Can you work these out from the model? Positions are in its coordinate system, mm. A direction names the side the tool comes from. Round coordinates to 2 decimals unless told otherwise and drop trailing zeros. Write each loop counter-clockwise with the first axis right and the second up, starting at its lowest first coordinate (ties: lowest second). Pieces come first, ordered by that corner, then holes. Notation, with made-up numbers: (62, 74) -> (74, 74) arc R21 ccw to (74, 88) -> close; hole circle Ø3 at (-8.5, 29). An arc over 180 degrees is marked (long way). Write item = value, one per line. Start each with the question number.
1) Imagine slicing it at D-D, the plane y = 44.5. Please give me the cut outline in (x, z), then the cut area to 3 significant figures.
2) I'm going to push flat-ended pins straight in: pin 1 (2.5 mm diameter, centred on y = 74.6, z = 10.5, fed in from -X); pin 2 (3.5 mm diameter, centred on x = 1, z = 10.5, fed in from -Y); pin 3 (4 mm diameter, centred on x = 0.5, y = 63, fed in from +Z); pin 4 (3 mm diameter, centred on y = 4, z = 3, fed in from -X). Where does each tip first touch, or does it pass through?
3) If I drill on line 1 (Y direction, x = 0.3, z = 10.5); line 2 (Z direction, x = -0.8, y = 74.6); line 3 (Z direction, x = -1.5, y = 35), over which ranges is the centre line in solid material (lowest first)?
4) Imagine slicing it at B-B, the plane y = 74.6. Please give me the cut outline in (x, z), then the cut area to 3 significant figures.
5) Imagine slicing it at A-A, the plane z = 10.5. Please give me the cut outline in (x, y).
6) Thinking about a two-plate mould opening in Y: for faces 4 (the face through (-2, 70, 11)), 5 (the face through (-0.03, 77.53, 7.6)), 6 (the face through (1.126, 5.082, 3.563)), 7 (the face through (0, 73, 10.9)), which applies, +Y half, -Y half, draft (parallel to the pull), parting line (faces both ways), or undercut?
7) Imagine slicing it at C-C, the plane y = 4. Please give me the cut outline in (x, z).
8) For faces 1 (the face through (0, 78.1, 11)), 2 (the face through (-2.42, 3.28, 0.73)), 3 (the face through (0, 64, 11)), which set-ups out of +Z, -Z, +X, -X, +Y, -Y let a thin tool reach every point of the face, with its end or its side?
from build123d import *

# Parameters (mm, degrees)
SKETCH1_W                                      = 7
SKETCH1_H                                      = 14
BOSS_EXTRUDE1_DEPTH                            = 70
CBORE_FOR_2_SOCKET_HEAD_CAP_SCREW1_D           = 2.4384
CBORE_FOR_2_SOCKET_HEAD_CAP_SCREW1_CBORE_D     = 4.7625
CBORE_FOR_2_SOCKET_HEAD_CAP_SCREW1_CBORE_DEPTH = 2.1844
CUT_EXTRUDE2_DEPTH                             = 71.696534569
LPATTERN1_COUNT                                = 3
LPATTERN1_PITCH                                = 2.5
LPATTERN1_COL_COUNT                            = 3
LPATTERN1_COL_PITCH                            = 2.5
FILLET1_R                                      = 0.2
CHAMFER1_SIZE                                  = 0.7
FILLET2_R                                      = 1
CUT_EXTRUDE4_DEPTH                             = 71.436141406
CUT_EXTRUDE4_DEPTH_BACK                        = 71.436141406
SKETCH6_W                                      = 1.5
SKETCH6_H                                      = 4
CHAMFER2_SIZE                                  = 0.5
FILLET4_R                                      = 0.5
SKETCH7_W                                      = 7
SKETCH7_H                                      = 14.1
BOSS_EXTRUDE2_DEPTH                            = 2
CUT_EXTRUDE5_REACH                             = 81.535
SKETCH9_R                                      = 1.65
FILLET5_R                                      = 2


with BuildPart() as part:
    # Sketch1 → Boss-Extrude1 (new body)
    with BuildSketch(Plane(origin=(0, 0, 0), x_dir=(1, 0, 0), z_dir=(0, 1, 0))):
        Rectangle(SKETCH1_W, SKETCH1_H)
    extrude(amount=BOSS_EXTRUDE1_DEPTH)

    # CBORE for #2 Socket Head Cap Screw1 (through all)
    with Locations(Plane(origin=(-3.5, 0, 0), x_dir=(0, 0, -1), z_dir=(-1, 0, 0))):
        with Locations((-3, -4), (3, -4)):
            CounterBoreHole(CBORE_FOR_2_SOCKET_HEAD_CAP_SCREW1_D / 2, CBORE_FOR_2_SOCKET_HEAD_CAP_SCREW1_CBORE_D / 2, CBORE_FOR_2_SOCKET_HEAD_CAP_SCREW1_CBORE_DEPTH)

    # Sketch4 → Cut-Extrude2 (cut, through all)
    with BuildSketch(Plane(origin=(3.5, 0, 0), x_dir=(0, 0, -1), z_dir=(1, 0, 0))):
        with BuildLine():
            Line((0.9, 220.888750438), (0.9, 70))
            ThreePointArc((0.9, 70), (0, 69.1), (-0.9, 70))
            Line((-0.9, 70), (-0.9, 220.888750438))
            Line((-0.9, 220.888750438), (-0.9, 522.666251314))
            Line((-0.9, 522.666251314), (0.9, 522.666251314))
            Line((0.9, 522.666251314), (0.9, 220.888750438))
        make_face()
    cut_extrude2 = extrude(amount=-CUT_EXTRUDE2_DEPTH, mode=Mode.SUBTRACT)

    # LPattern1: Cut-Extrude2 ×3
    with Locations(*[(0, 0, i * LPATTERN1_PITCH) for i in range(1, LPATTERN1_COUNT)]):
        add(cut_extrude2, mode=Mode.SUBTRACT)

    # LPattern1 col: Cut-Extrude2 ×3
    with Locations(*[(0, 0, -i * LPATTERN1_COL_PITCH) for i in range(1, LPATTERN1_COL_COUNT)]):
        add(cut_extrude2, mode=Mode.SUBTRACT)

    # Fillet1
    fillet1_edges = [part.edges().sort_by_distance(p)[0] for p in [
        (0, 70, -0.9),
        (0, 70, 0.9),
        (3.5, 69.1, 0),
        (-3.5, 69.1, 0),
        (0, 70, -3.4),
        (0, 70, -1.6),
        (3.5, 69.1, -2.5),
        (-3.5, 69.1, -2.5),
        (0, 70, -5.9),
        (0, 70, -4.1),
        (3.5, 69.1, -5),
        (-3.5, 69.1, -5),
        (0, 70, 1.6),
        (0, 70, 3.4),
        (3.5, 69.1, 2.5),
        (-3.5, 69.1, 2.5),
        (0, 70, 4.1),
        (0, 70, 5.9),
        (3.5, 69.1, 5),
        (-3.5, 69.1, 5),
    ]]
    fillet(fillet1_edges, radius=FILLET1_R)

    # Chamfer1
    chamfer1_edges = [part.edges().sort_by_distance(p)[0] for p in [
        (0, 70, -7),
    ]]
    chamfer(chamfer1_edges, length=CHAMFER1_SIZE)

    # Fillet2
    # the kernel refuses this fillet: 1 mm, written as the material it takes off along each edge
    with BuildSketch(Plane(origin=(-4.535533906, 69.3, -7), x_dir=(0, 0.707106781186555, 0.70710678118654), z_dir=(1, 0, 0))) as fillet2_piece_1:
        with BuildLine():
            CenterArc((FILLET2_R * 0.414213562373, FILLET2_R), FILLET2_R, 225, 45)
            Line((-FILLET2_R * 0.292893218813, FILLET2_R * 0.292893218813), (-FILLET2_R * 0.307035354437, FILLET2_R * 0.27875108319))
            Line((-FILLET2_R * 0.307035354437, FILLET2_R * 0.27875108319), (-FILLET2_R * 0.00828427124746, -FILLET2_R * 0.02))
            Line((-FILLET2_R * 0.00828427124746, -FILLET2_R * 0.02), (FILLET2_R * 0.414213562373, -FILLET2_R * 0.02))
            Line((FILLET2_R * 0.414213562373, -FILLET2_R * 0.02), (FILLET2_R * 0.414213562373, 0))
        make_face()
    extrude(amount=9.071067812, mode=Mode.SUBTRACT)
    with BuildSketch(Plane(origin=(-4.448522012, 70, -6.3), x_dir=(0, 0, 1), z_dir=(1, 0, 0))) as fillet2_piece_2:
        with BuildLine():
            CenterArc((0.438824243, 0.97538932), FILLET2_R, 225, 32.262207343)
            Line((-0.268282539, 0.268282539), (-0.282424674, 0.254140403))
            Line((-0.282424674, 0.254140403), (-0.014142136, -0.014142136))
            Line((-0.014142136, -0.014142136), (0, -0.02))
            ThreePointArc((0, -0.02), (0.109167309, -0.02), (0.213924825, -0.019507786))
            Line((0.213924825, -0.019507786), (0.218334617, 0))
        make_face()
    extrude(amount=8.897044023, mode=Mode.SUBTRACT)

    # Sketch6 → Cut-Extrude4 (cut, two sides: drawn at the far end of the back side and taken through both)
    with BuildSketch(Plane(origin=(0, 0, 0), x_dir=(0, 0, -1), z_dir=(1, 0, 0)).offset(-CUT_EXTRUDE4_DEPTH_BACK)):
        with Locations((6.25, 65)):
            Rectangle(SKETCH6_W, SKETCH6_H)
    extrude(amount=CUT_EXTRUDE4_DEPTH + CUT_EXTRUDE4_DEPTH_BACK, mode=Mode.SUBTRACT)

    # Chamfer2
    chamfer2_edges = [part.edges().sort_by_distance(p)[0] for p in [
        (0, 67, -7),
    ]]
    chamfer(chamfer2_edges, length=CHAMFER2_SIZE)

    # Fillet4
    fillet4_edges = [part.edges().sort_by_distance(p)[0] for p in [
        (0, 63, -7),
        (0, 63, -5.5),
        (0, 67.5, -7),
        (0, 67, -6.5),
    ]]
    fillet(fillet4_edges, radius=FILLET4_R)

    # Sketch7 → Boss-Extrude2 (add, symmetric)
    with BuildSketch(Plane(origin=(0, 0, 0), x_dir=(0, 0, -1), z_dir=(1, 0, 0))):
        with Locations((-10.5, 71.05)):
            Rectangle(SKETCH7_W, SKETCH7_H)
    extrude(amount=BOSS_EXTRUDE2_DEPTH, both=True)

    # Sketch9 → Cut-Extrude5 (cut, up to next)
    with BuildSketch(Plane(origin=(2, 0, 0), x_dir=(0, 0, -1), z_dir=(1, 0, 0)), mode=Mode.PRIVATE) as cut_extrude5_sk1:
        with Locations((-10.5, 74.6)):
            Circle(SKETCH9_R)
    cut_extrude5_tool1 = extrude(cut_extrude5_sk1.sketch, amount=-CUT_EXTRUDE5_REACH, mode=Mode.PRIVATE) & part.part
    add(cut_extrude5_tool1.solids().sort_by_distance((2, 74.6, 10.5))[0], mode=Mode.SUBTRACT)

    # Fillet5
    fillet5_edges = [part.edges().sort_by_distance(p)[0] for p in [
        (0, 78.1, 7),
        (0, 64, 7),
        (0, 64, 14),
        (0, 78.1, 14),
    ]]
    fillet(fillet5_edges, radius=FILLET5_R)


solid = part.part
Reported:
q1.outline = (-3.5, -7) -> (3.5, -7) -> (3.5, 7) -> (-3.5, 7) -> close
q1.area = 98.0 mm²
q2.pin_1 = through
q2.pin_2 = 63.98
q2.pin_3 = 13.73
q2.pin_4 = -1.32
q3.line_1 = 64 to 72.95, 76.25 to 78.1
q3.line_2 = 7 to 8.85, 12.15 to 14
q3.line_3 = -7 to 7
q4.outline = (-2, 7) -> (2, 7) -> (2, 8.85) -> (-2, 8.85) -> close; (-2, 12.15) -> (2, 12.15) -> (2, 14) -> (-2, 14) -> close
q4.area = 14.8 mm²
q5.outline = (-2, 64) -> (2, 64) -> (2, 72.95) -> (-2, 72.95) -> close; (-2, 76.25) -> (2, 76.25) -> (2, 78.1) -> (-2, 78.1) -> close
q6.face_4 = draft
q6.face_5 = +Y half
q6.face_6 = undercut
q6.face_7 = undercut
q7.outline = (-3.5, -7) -> (3.5, -7) -> (3.5, -4.22) -> (-1.32, -4.22) -> (-1.32, -5.38) -> (-3.5, -5.38) -> close; (-3.5, -0.62) -> (-1.32, -0.62) -> (-1.32, -1.78) -> (3.5, -1.78) -> (3.5, 1.78) -> (-1.32, 1.78) -> (-1.32, 0.62) -> (-3.5, 0.62) -> close; (-3.5, 5.38) -> (-1.32, 5.38) -> (-1.32, 4.22) -> (3.5, 4.22) -> (3.5, 7) -> (-3.5, 7) -> close
q8.face_1 = +Z, -Z, +X, -X, +Y
q8.face_2 = -X
q8.face_3 = +Z, +X, -X, -Y
